Read the model definition and answer for the solid it produces. Units are mm, in the model's axes. A direction names the side the tool comes from. Coordinates: 2 decimals unless noted, no trailing zeros. Order: outer loops, then holes, each group sorted by start corner. A loop starts at its lowest first (then second) coordinate and runs counter-clockwise, first axis right, second up. Notation, with made-up numbers: (-27, -22.75) -> (-2, -22.75) arc R23 cw to (-2, 14.25) -> close; hole circle Ø5 at (44.25, 39.5). An arc over 180 degrees is marked (long way). Return JSON: item names as keys, results as strings. Group by question number.
```python
from build123d import *

# Parameters (mm, degrees)
BOSS_EXTRUDE1_DEPTH = 1
FILLET1_R           = 0.75


with BuildPart() as part:
    # Sketch1 → Boss-Extrude1 (new body)
    with BuildSketch(Plane(origin=(0, 0, 0), x_dir=(1, 0, 0), z_dir=(0, 1, 0))):
        with BuildLine():
            ThreePointArc((2.764713205, -21.975), (15.303300859, -25.303300859), (11.975, -12.764713205))
            Line((11.975, -12.764713205), (11.975, -7.235286795))
            ThreePointArc((11.975, -7.235286795), (17.5, 0), (11.975, 7.235286795))
            Line((11.975, 7.235286795), (11.975, 21.975))
            Line((11.975, 21.975), (-2.764713205, 21.975))
            ThreePointArc((-2.764713205, 21.975), (-15.238556982, 25.367263805), (-12.15, 12.814772098))
            Line((-12.15, 12.814772098), (-12.15, 7.185227902))
            ThreePointArc((-12.15, 7.185227902), (-17.494366614, 0.290635598), (-12.7, -6.997142274))
            Line((-12.7, -6.997142274), (-12.7, -13.002857726))
            ThreePointArc((-12.7, -13.002857726), (-15.02663315, -25.566233841), (-2.764713205, -21.975))
            Line((-2.764713205, -21.975), (2.764713205, -21.975))
        make_face()
        with BuildLine():
            Line((8.025, -7.235286795), (8.025, -12.764713205))
            ThreePointArc((8.025, -12.764713205), (4.696699141, -14.696699141), (2.764713205, -18.025))
            Line((2.764713205, -18.025), (-2.764713205, -18.025))
            ThreePointArc((-2.764713205, -18.025), (-4.433766159, -14.97336685), (-7.3, -13.002857726))
            Line((-7.3, -13.002857726), (-7.3, -6.997142274))
            ThreePointArc((-7.3, -6.997142274), (-4.621848486, -5.22737853), (-2.928932188, -2.5))
            Line((-2.928932188, -2.5), (2.928932188, -2.5))
            ThreePointArc((2.928932188, -2.5), (4.894750646, -5.494217781), (8.025, -7.235286795))
        make_face(mode=Mode.SUBTRACT)
        with BuildLine():
            Line((8.025, 18.025), (8.025, 7.235286795))
            ThreePointArc((8.025, 7.235286795), (4.894750646, 5.494217781), (2.928932188, 2.5))
            Line((2.928932188, 2.5), (-2.928932188, 2.5))
            ThreePointArc((-2.928932188, 2.5), (-4.828456418, 5.431863122), (-7.85, 7.185227902))
            Line((-7.85, 7.185227902), (-7.85, 12.814772098))
            ThreePointArc((-7.85, 12.814772098), (-4.632736195, 14.761443018), (-2.764713205, 18.025))
            Line((-2.764713205, 18.025), (8.025, 18.025))
        make_face(mode=Mode.SUBTRACT)
    extrude(amount=BOSS_EXTRUDE1_DEPTH)

    # Fillet1
    fillet1_edges = [part.edges().sort_by_distance(p)[0] for p in [
        (2.764713205, 0.5, 18.025),
        (-2.764713205, 0.5, 18.025),
        (-2.764713205, 0.5, 21.975),
        (2.764713205, 0.5, 21.975),
        (11.975, 0.5, 12.764713205),
        (11.975, 0.5, 7.235286795),
        (8.025, 0.5, 7.235286795),
        (8.025, 0.5, 12.764713205),
        (-2.928932188, 0.5, 2.5),
        (2.928932188, 0.5, 2.5),
        (2.928932188, 0.5, -2.5),
        (-2.928932188, 0.5, -2.5),
        (11.975, 0.5, -7.235286795),
        (11.975, 0.5, -21.975),
        (-2.764713205, 0.5, -21.975),
        (-2.764713205, 0.5, -18.025),
        (8.025, 0.5, -18.025),
        (8.025, 0.5, -7.235286795),
        (-12.15, 0.5, -12.814772098),
        (-12.15, 0.5, -7.185227902),
        (-7.85, 0.5, -7.185227902),
        (-7.85, 0.5, -12.814772098),
        (-12.7, 0.5, 13.002857726),
        (-12.7, 0.5, 6.997142274),
        (-7.3, 0.5, 6.997142274),
        (-7.3, 0.5, 13.002857726),
    ]]
    fillet(fillet1_edges, radius=FILLET1_R)


solid = part.part
```
1. Find section C-C on x = 13.5. Determine the outline of the cut face in (y, z).
2. Find section B-B on z = 8.5. Determine the outline of the cut face in (x, y) (3 decimals), and give its area (3 significant figures).
3. Which of the six approach directions +Z, -Z, +X, -X, +Y, -Y give full straight-line access (tool end or side, diameter ignored) to faces 1 (the face through (4.9, 0.5, -5.5)), 2 (the face through (-12.7, 0.5, 10)), 3 (the face through (11.975, 0.5, -14.4))?
4. For a pull along X with two mould halves and no side action, classify faces 4 (the face through (11.975, 0.5, 10)), 5 (the face through (-7.85, 0.5, -10)), 6 (the face through (-17.49, 0.49, -0.39)) as released by +X, released by -X, zero draft, split by the parting line, or undercut.
5. Given pin 1 (0.5 mm diameter, centred on y = 0.5, z = -11, fed in from +X) (3 decimals); pin 2 (0.5 mm diameter, centred on y = 0.5, z = 9.5, fed in from -X); pin 3 (0.5 mm diameter, centred on x = 3.5, y = 0.5, fed in from -Z) (3 decimals); pin 4 (3 mm diameter, centred on x = 4, z = 8, fed in from -Y), each flat-ended and moving along its own axis, determine where each tip first touches the part or whether it passes through.
6. Straight lines are drawn through the part: L1, parallel to Z at x = 0.5, y = 0.2 (3 decimals); L2, parallel to X at y = 0.3, z = 12 (3 decimals); L3, parallel to Z at x = -13, y = 0.6. For each, find the intervals that lie inside material, in ascending order.
7. Find section A-A on x = 1.5. Determine the outline of the cut face in (y, z) (3 decimals).
8. Find section D-D on y = 0.6. Give the number of separate pieces and of enclosed holes in the cut face, and give its area (3 significant figures).
Result:
{
 "1": {"outline": "(0, -6.63) -> (1, -6.63) -> (1, 6.63) -> (0, 6.63) -> close; (0, 13.37) -> (1, 13.37) -> (1, 26.63) -> (0, 26.63) -> close"},
 "2": {"outline": "(-12.7, 0) -> (-7.3, 0) -> (-7.3, 1) -> (-12.7, 1) -> close; (8.025, 0) -> (11.975, 0) -> (11.975, 1) -> (8.025, 1) -> close", "area": "9.35 mm^2"},
 "3": {"face 1": "+Y, -Y", "face 2": "-X, +Y, -Y", "face 3": "-Z, +X, +Y, -Y"},
 "4": {"face 4": "released by +X", "face 5": "undercut", "face 6": "released by -X"},
 "5": {"pin 1": "x = 11.975", "pin 2": "x = -12.7", "pin 3": "z = -21.975", "pin 4": "through"},
 "6": {"L1": "-21.975 to -18.025, -2.5 to 2.5, 18.025 to 21.975", "L2": "-12.7 to -7.3, 8.025 to 11.975", "L3": "-26.87 to -13.13, -6.87 to 6.89, 13.11 to 26.87"},
 "7": {"outline": "(0, -21.975) -> (1, -21.975) -> (1, -18.025) -> (0, -18.025) -> close; (0, -2.5) -> (1, -2.5) -> (1, 2.5) -> (0, 2.5) -> close; (0, 18.025) -> (1, 18.025) -> (1, 21.975) -> (0, 21.975) -> close"},
 "8": {"separate pieces": "1", "enclosed holes": "2", "area": "1,100 mm^2"}
}
